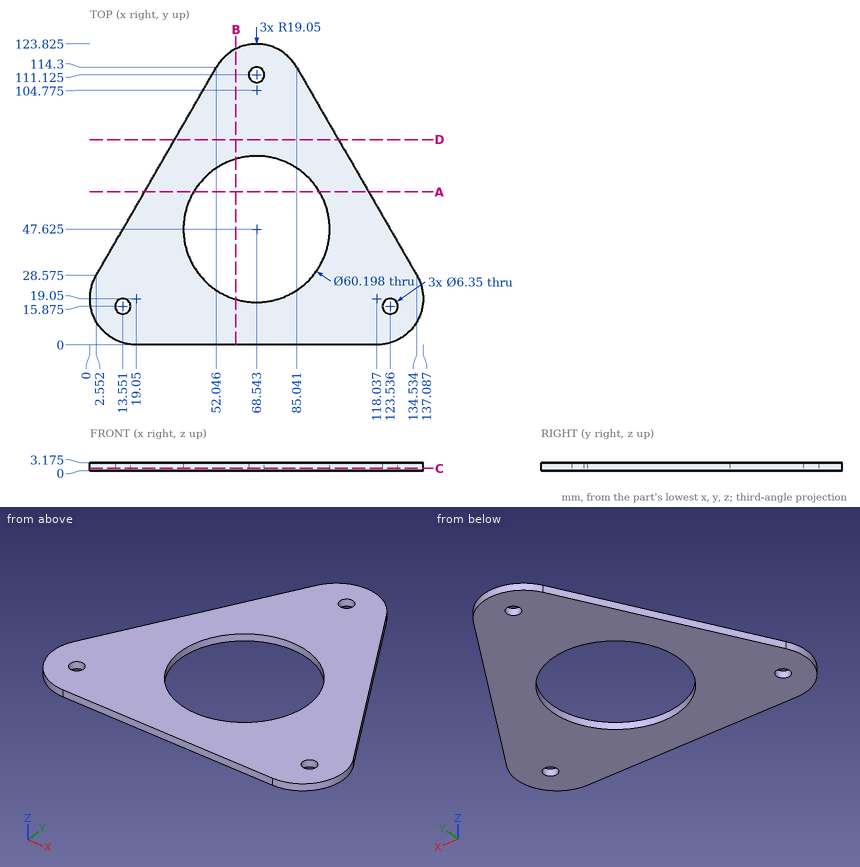
Study the drawing (mm; zero at the part's minimum x, y, z) and answer. Round coordinates to 2 decimals unless told otherwise and drop trailing zeros. Write each loop counter-clockwise with the first axis right and the second up, starting at its lowest first coordinate (ties: lowest second). Pieces come first, ordered by that corner, then holes. Notation, with made-up numbers: (76.25, 40.5) - (111.25, 40.5) arc R26 cw to (111.25, 68.5) - close; hole circle Ø3 at (61.25, -25.5). An arc over 180 degrees is marked (long way). Return JSON: item names as keys, results as strings. Group by question number.
Q1. The part is cut by section B-B on x = 60. Write down the section's boundary in (y, z) (1 decimal).
Q2. The part is cut by section C-C on z = 0.9. Count the separate pieces of the cut face and the enclosed holes in it, then the cut area to 3 significant figures.
Q3. Find the intervals of material crossed by L1, parallel to Y at x = 94, z = 1.1 (1 decimal); L2, parallel to X at y = 42.5, z = 1.6 (1 decimal); L3, parallel to Y at x = 53.5, z = 2.6 (1 decimal), in increasing order.
Q4. The part is cut by section A-A on y = 63. Write down the section's boundary in (x, z) (1 decimal).
Q5. Each of these flat-tipped pins is pushed along its axis until it touches: pin 1 Ø1.5 at (y, z) = (52.5, 2.5) entering from +X (1 decimal); pin 2 Ø4 at (x, y) = (13.55, 15.88) entering from -Z. Where does it stop, or does it pass through?
Q6. The part is cut by section D-D on y = 84.5. Write down the section's boundary in (x, z) (1 decimal).
Solved:
{
 "1": {"outline": "(0, 0) - (18.8, 0) - (18.8, 3.2) - (0, 3.2) - close; (76.5, 0) - (121.8, 0) - (121.8, 3.2) - (76.5, 3.2) - close"},
 "2": {"separate pieces": "1", "enclosed holes": "4", "area": "8,100 mm²"},
 "3": {"L1": "0 to 31.6, 63.7 to 98.8", "L2": "10.6 to 38.9, 98.2 to 126.5", "L3": "0 to 21.6, 73.7 to 116.5"},
 "4": {"outline": "(22.4, 0) - (42.7, 0) - (42.7, 3.2) - (22.4, 3.2) - close; (94.4, 0) - (114.7, 0) - (114.7, 3.2) - (94.4, 3.2) - close"},
 "5": {"pin 1": "x = 121.2", "pin 2": "through"},
 "6": {"outline": "(34.8, 0) - (102.2, 0) - (102.2, 3.2) - (34.8, 3.2) - close"}
}
